Answer from the drawing. Dimensions are ordinates in mm from the lowest x, y and z of the part. A direction names the side the tool comes from. Round coordinates to 2 decimals unless told otherwise and drop trailing zeros. Write each loop counter-clockwise with the first axis right and the second up, starting at its lowest first coordinate (ties: lowest second). Pieces come first, ordered by that corner, then holes. Notation, with made-up numbers: (-20.5, 12.25) - (-10.5, 12.25) arc R25 cw to (-10.5, 27.25) - close; hole circle Ø7 at (28, 43). An arc over 180 degrees is marked (long way). Answer in a Markdown table with one row per item.
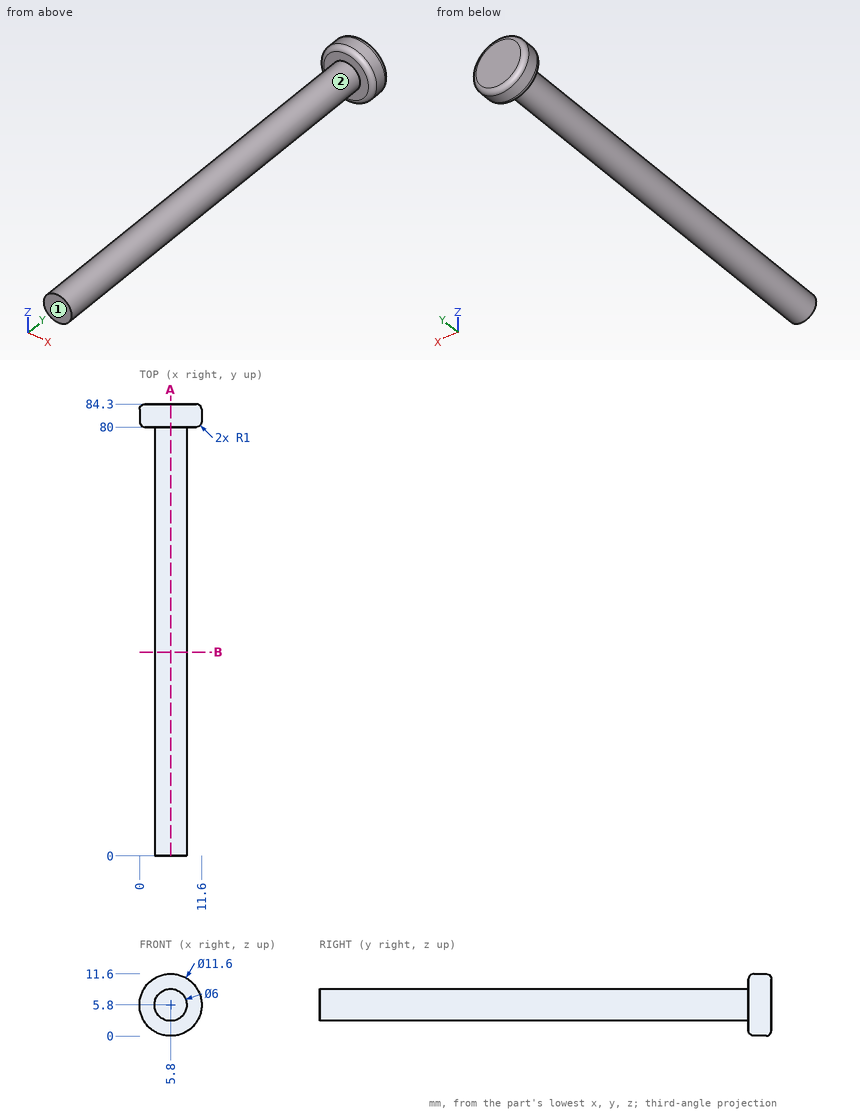
(1) For the marked faces 1 and 2, determine the directions among +Z, -Z, +X, -X, +Y, -Y from which every point of the face is accessible in a straight line to the end or side of a thin tool.
Checked values:
| item | result |
|---|---|
| face 1 | +Z, -Z, +X, -X, -Y |
| face 2 | -Y |
(2) Flat-ended cylindrical pins translate along their axes: pin 1 (5 mm diameter, centred on x = 1, y = 20.5, fed in from +Z); pin 2 (1 mm diameter, centred on x = 4, y = 32.5, fed in from +Z); pin 3 (6 mm diameter, centred on x = 7.5, y = 18, fed in from -Z). Find the tip coordinate at first contact, or state that the pin passes through.
Checked values:
| item | result |
|---|---|
| pin 1 | stops at z = 7.73 |
| pin 2 | stops at z = 8.5 |
| pin 3 | stops at z = 2.8 |
(3) Section B-B (y = 38) is taken. Give the vertices of the cut face in (x, z), and give its area (3 significant figures).
Checked values:
| item | result |
|---|---|
| outline | circle Ø6 at (5.8, 5.8) |
| area | 28.3 mm2 |
(4) Find the intervals of material crossed by line 1 (Y direction, x = 10.25, z = 7.5); line 2 (Z direction, x = 6, y = 72.5); line 3 (Y direction, x = 1.25, z = 2.5), in increasing order.
Checked values:
| item | result |
|---|---|
| line 1 | y = 80 to 84.3 |
| line 2 | z = 2.81 to 8.79 |
| line 3 | y = 80.43 to 83.87 |
(5) Section A-A (x = 5.8) is taken. Give the vertices of the cut face in (y, z), and give its area (3 significant figures).
Checked values:
| item | result |
|---|---|
| outline | (0, 2.8) - (80, 2.8) - (80, 1) arc R1 ccw to (81, 0) - (83.3, 0) arc R1 ccw to (84.3, 1) - (84.3, 10.6) arc R1 ccw to (83.3, 11.6) - (81, 11.6) arc R1 ccw to (80, 10.6) - (80, 8.8) - (0, 8.8) - close |
| area | 529 mm2 |
